```python
from build123d import *

# Parameters (mm, degrees)
F0_W     = 24.9907784164
F0_H     = 38.2269993424
F1_DEPTH = 38.1
F2_W     = 12.2484434396
F2_H     = 7.2107780725
F3_DEPTH = 24.9917784164
F5_DEPTH = 24.9917784164


with BuildPart() as f1:
    # F0 (on Right) → F1 (new body)
    with BuildSketch(Plane.YZ):
        with Locations((12.4953892082, 19.1134996712)):
            Rectangle(F0_W, F0_H)
    extrude(amount=F1_DEPTH)

    # F2 (on face) → F3 (cut, through all)
    with BuildSketch(Plane.XZ):
        with Locations((18.471444957, 3.6053890362)):
            Rectangle(F2_W, F2_H)
    extrude(amount=-F3_DEPTH, mode=Mode.SUBTRACT)

    # F4 (on face) → F5 (cut, through all)
    with BuildSketch(Plane.XZ):
        Polygon((0, 0), (15.113000758, 38.2269993424), (0, 38.2269993424), align=None)
        Polygon((38.1, 38.2269993424), (23.8054450601, 38.2269993424), (38.1, 0), align=None)
    extrude(amount=-F5_DEPTH, mode=Mode.SUBTRACT)


solid = f1.part
```
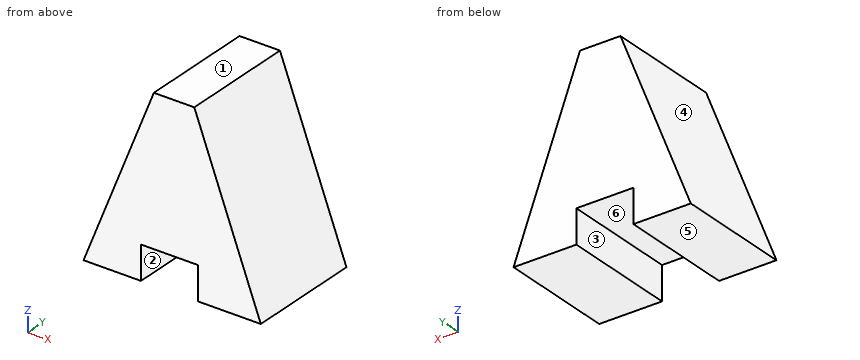
The listing builds one solid part. Answer for the finished solid, in the listing's coordinates (mm). Face numbers are marked on the shaded views. A direction names the side the tool comes from. Coordinates: 2 decimals unless noted, no trailing zeros. Order: outer loops, then holes, each group sorted by start corner. A loop starts at its lowest first (then second) coordinate and runs counter-clockwise, first axis right, second up. Notation, with made-up numbers: M -18,-27 L 3,-27 A16 ccw 3,-3 Z; hole C -0.5,58.5 d4. An arc over 180 degrees is marked long. Answer as a JSON object with one key per item and string values. Group by question number.
1. A tool of negligible diameter and unlimited length cuts with its end or side. For the marked faces 1 and 2, from which of +Z, -Z, +X, -X, +Y, -Y can it reach the whole face along a straight path? Write none if from no direction.
2. Section D-D on z = 15 is taken. Write down the section's boundary in (x, y).
3. Straight lines are drawn through the part: line 1 (X direction, y = 6.5, z = 3.5); line 2 (X direction, y = 22.75, z = 12); line 3 (X direction, y = 17.75, z = 5.5). For each, find the intervals that lie inside material, in ascending order.
4. Flat-ended cylindrical pins translate along their axes: P1, Ø1.5, axis at y = 9.5, z = 21.5, coming from the +X side; P2, Ø1.5, axis at x = 4.5, z = 14.5, coming from the +Y side; P3, Ø1.5, axis at y = 15.5, z = 27, coming from the +X side; P4, Ø6, axis at y = 4, z = 22, coming from the -X side. Find the tip coordinate at first contact, or state that the pin passes through.
5. Section A-A on z = 3 is taken. Write down the section's boundary in (x, y).
6. Determine the mould class of the marked faces 3, 4, 5 and 6 for opening direction X: released by +X, released by -X, zero draft, split by the parting line, or undercut.
7. Section B-B on y = 3.25 is taken. Write down the section's boundary in (x, z).
8. Section C-C on x = 8.5 is taken. Write down the section's boundary in (y, z), then the cut area to 3 significant figures.
Values follow:
{
 "1": {"face 1": "+Z, +X, -X, +Y, -Y", "face 2": "-Z, +Y, -Y"},
 "2": {"outline": "M 5.93,0 L 32.49,0 L 32.49,24.99 L 5.93,24.99 Z"},
 "3": {"line 1": "1.38 to 12.35, 24.6 to 36.79", "line 2": "4.74 to 33.61", "line 3": "2.17 to 12.35, 24.6 to 36.04"},
 "4": {"P1": "x = 30.34", "P2": "through", "P3": "x = 28.28", "P4": "x = 7.51"},
 "5": {"outline": "M 1.19,0 L 12.35,0 L 12.35,24.99 L 1.19,24.99 Z; M 24.6,0 L 36.98,0 L 36.98,24.99 L 24.6,24.99 Z"},
 "6": {"face 3": "undercut", "face 4": "released by -X", "face 5": "zero draft", "face 6": "undercut"},
 "7": {"outline": "M 0,0 L 12.35,0 L 12.35,7.21 L 24.6,7.21 L 24.6,0 L 38.1,0 L 23.81,38.23 L 15.11,38.23 Z"},
 "8": {"outline": "M 0,0 L 24.99,0 L 24.99,21.5 L 0,21.5 Z", "area": "537 mm2"}
}
